Verification items for the finished model (mm, model axes). A direction names the side the tool comes from. Give positions to 0.01 mm unless a question says otherwise; leave off trailing zeros. Loops run counter-clockwise (first coordinate to the right, second up) from the corner with the lowest first, then second, coordinate; pieces in that order, holes last. Notation, with made-up numbers: M 80.5,32 L 139.5,32 A19 ccw 139.5,53 Z; hole C 15,28 d2. An arc over 180 degrees is marked long. Use a Markdown table: item, result.
from build123d import *

# Parameters (mm, degrees)
SKETCH1_R           = 17.326400039
BOSS_EXTRUDE1_DEPTH = 30
SKETCH3_W           = 16.12994251
SKETCH3_H           = 14.480289299
BOSS_EXTRUDE2_DEPTH = 80
SKETCH4_W           = 11.547572479
SKETCH4_H           = 8.79815046
BOSS_EXTRUDE3_DEPTH = 80
SKETCH5_R           = 5.135526513
BOSS_EXTRUDE4_DEPTH = 162


with BuildPart() as part:
    # Sketch1 → Boss-Extrude1 (new body)
    with BuildSketch(Plane.XY):
        with BuildLine():
            Line((19.721500067, 11.745451968), (163.015891701, 11.745451968))
            Line((163.015891701, 11.745451968), (163.015891701, -11.745451968))
            Line((163.015891701, -11.745451968), (19.721500067, -11.745451968))
            ThreePointArc((19.721500067, -11.745451968), (-22.954154456, 0), (19.721500067, 11.745451968))
        make_face()
        Circle(SKETCH1_R, mode=Mode.SUBTRACT)
    extrude(amount=BOSS_EXTRUDE1_DEPTH)

    # Sketch3 → Boss-Extrude2 (add)
    with BuildSketch(Plane(origin=(0, 11.745451968, 0), x_dir=(1, 0, 0), z_dir=(0, 1, 0))):
        with Locations((146.281505943, -15.733179206)):
            Rectangle(SKETCH3_W, SKETCH3_H)
    boss_extrude2 = extrude(amount=BOSS_EXTRUDE2_DEPTH)

    # Sketch4 → Boss-Extrude3 (add)
    with BuildSketch(Plane(origin=(0, 0, 8.493034556), x_dir=(-1, 0, 0), z_dir=(0, 0, -1))):
        with Locations((-146.556448146, 84.160187296)):
            Rectangle(SKETCH4_W, SKETCH4_H)
    boss_extrude3 = extrude(amount=BOSS_EXTRUDE3_DEPTH)

    # Mirror1: Boss-Extrude2, Boss-Extrude3 across plane
    add(boss_extrude2.mirror(Plane.ZX))
    add(boss_extrude3.mirror(Plane.ZX))

    # Sketch5 → Boss-Extrude4 (add)
    with BuildSketch(Plane(origin=(0, -79.761112066, 0), x_dir=(1, 0, 0), z_dir=(0, 1, 0))):
        with Locations(Location((146.648095546, 63.736113616, 0), (0, 0, 270))):
            Circle(SKETCH5_R)
    extrude(amount=BOSS_EXTRUDE4_DEPTH)


solid = part.part
(1) Set-up check for faces 5 (the flat face through (154.346, 51, 16)), 6 (the flat face through (146, -91.745, 16)), 7 (the flat face through (147, 88.559, -31)): record each of +Z, -Z, +X, -X, +Y, -Y from which the full face is reachable in a straight line by a thin tool's end or side.
Results below:
| item | result |
|---|---|
| face 5 | +Z, -Z, +X, +Y |
| face 6 | +Z, -Z, +X, -X, -Y |
| face 7 | -Z, +X, -X, +Y |
(2) Cross-section at B-B on x = 0. Record the cut outline in (y, z).
Results below:
| item | result |
|---|---|
| outline | M -22.95,0 L -17.33,0 L -17.33,30 L -22.95,30 Z; M 17.33,0 L 22.95,0 L 22.95,30 L 17.33,30 Z |
(3) Cross-section at A-A on z = -13.5. Record the cut outline in (x, y).
Results below:
| item | result |
|---|---|
| outline | M 140.78,-88.56 L 152.33,-88.56 L 152.33,-79.76 L 140.78,-79.76 Z; M 140.78,79.76 L 152.33,79.76 L 152.33,88.56 L 140.78,88.56 Z |
(4) Cross-section at C-C on y = 46.5. Record the cut outline in (x, z).
Results below:
| item | result |
|---|---|
| outline | M 138.22,8.49 L 154.35,8.49 L 154.35,22.97 L 138.22,22.97 Z; C 146.65,-63.74 d10.27 |
(5) Draft check along Y on faces 1 (the flat face through (147, 79.761, -31)), 2 (the cylindrical face through (-13.75, -10.54, 14.79)), 3 (the flat face through (71, 0, 30)), 4 (the flat face through (147, -88.559, -31)). Enter one of: +Y half, -Y half, draft (parallel to the pull), parting line (faces both ways), or undercut.
Results below:
| item | result |
|---|---|
| face 1 | undercut |
| face 2 | undercut |
| face 3 | draft |
| face 4 | -Y half |
(6) Cross-section at D-D on z = 20. Record the cut outline in (x, y).
Results below:
| item | result |
|---|---|
| outline | M 19.72,-11.75 L 138.22,-11.75 L 138.22,-91.75 L 154.35,-91.75 L 154.35,-11.75 L 163.02,-11.75 L 163.02,11.75 L 154.35,11.75 L 154.35,91.75 L 138.22,91.75 L 138.22,11.75 L 19.72,11.75 A22.95 ccw long Z; hole C 0,0 d34.65 |
(7) Material ranges on line 1 (Y direction, x = 0, z = 6); line 2 (Y direction, x = 143.5, z = -13); line 3 (Y direction, x = 85, z = 6.5), recorded low to high.
Results below:
| item | result |
|---|---|
| line 1 | -22.95 to -17.33, 17.33 to 22.95 |
| line 2 | -88.56 to -79.76, 79.76 to 88.56 |
| line 3 | -11.75 to 11.75 |
(8) Gauge pin test, flat ends, axial feed: P1, Ø4.5, axis at y = 85.5, z = -40, coming from the -X side; P2, Ø8, axis at x = 147.5, y = 56, coming from the -Z side; P3, Ø6, axis at x = 146.5, z = -31.5, coming from the +Y side. Record the tip position at first contact, or that the pin passes through.
Results below:
| item | result |
|---|---|
| P1 | x = 140.78 |
| P2 | z = -68.87 |
| P3 | y = 88.56 |
